The model under review builds one solid part; all positions refer to its coordinate system, in mm. A direction names the side the tool comes from. Coordinates: 2 decimals unless noted, no trailing zeros. Write each question's results on one line, items separated by ' | '.
```python
from build123d import *

# Parameters (mm, degrees)
F0_W          = 60
F0_H          = 40
F1_DEPTH      = 25
F1_TAPER      = 5
F1_DEPTH_BACK = 25
F1_TAPER_BACK = 5
F2_R          = 7.5
F3_DEPTH      = 45


with BuildPart() as f1:
    # F0 (on Top) → F1 (new body, two sides)
    with BuildSketch(Plane.XY) as f1_sk:
        with Locations((30, 20)):
            Rectangle(F0_W, F0_H)
    extrude(amount=F1_DEPTH, taper=F1_TAPER)
    extrude(f1_sk.sketch, amount=-F1_DEPTH_BACK, taper=F1_TAPER_BACK)

    # F2 (on face) → F3 (cut)
    with BuildSketch(Plane.XY.offset(25)):
        with Locations((30, 20)):
            Circle(F2_R)
    extrude(amount=-F3_DEPTH, mode=Mode.SUBTRACT)


solid = f1.part
```
Q1. Clearance check with flat-ended pins moving along their axes: P1, Ø3, axis at y = 16.5, z = 18.5, coming from the -X side; P2, Ø7.5, axis at x = 31, y = 18, coming from the +Z side; P3, Ø2, axis at x = 46.5, z = -2, coming from the +Y side; P4, Ø4, axis at y = 34.5, z = -2, coming from the +X side. State where each tip first meets the part, or that it passes through.
Solution:
P1: x = 1.49 | P2: z = -20 | P3: y = 39.91 | P4: x = 60
Q2. Machinability: for faces 1 (the flat face through (1.08, 19.72, 12.33)), 2 (the cylindrical face through (24.5, 25.1, 2.8)), which of the approach directions +Z, -Z, +X, -X, +Y, -Y give a long, thin tool a straight path to every point of the face, cutting with its end or side? Answer none if there is none.
Solution:
face 1: +Z, -X, +Y, -Y | face 2: +Z
Q3. Draft analysis for pull direction Y (two halves, no side actions). For faces 3 (the flat face through (58.92, 20.28, 12.33)), 4 (the flat face through (29.58, 38.92, 12.33)), 5 (the flat face through (30, 20, -20)), state which applies: pulls with the +Y half, pulls with the -Y half, needs draft (parallel to the pull), parting line crosses it, or undercut.
Solution:
face 3: needs draft | face 4: pulls with the +Y half | face 5: undercut
Q4. For line 1 (X direction, y = 24.5, z = 11); line 2 (Y direction, x = 30, z = -1); line 3 (X direction, y = 26, z = -13), list the stretches that pass through material, from the lowest coordinate up. Write a range as from..to.
Solution:
line 1: 0.96..24, 36..59.04 | line 2: 0.09..12.5, 27.5..39.91 | line 3: 1.14..25.5, 34.5..58.86
